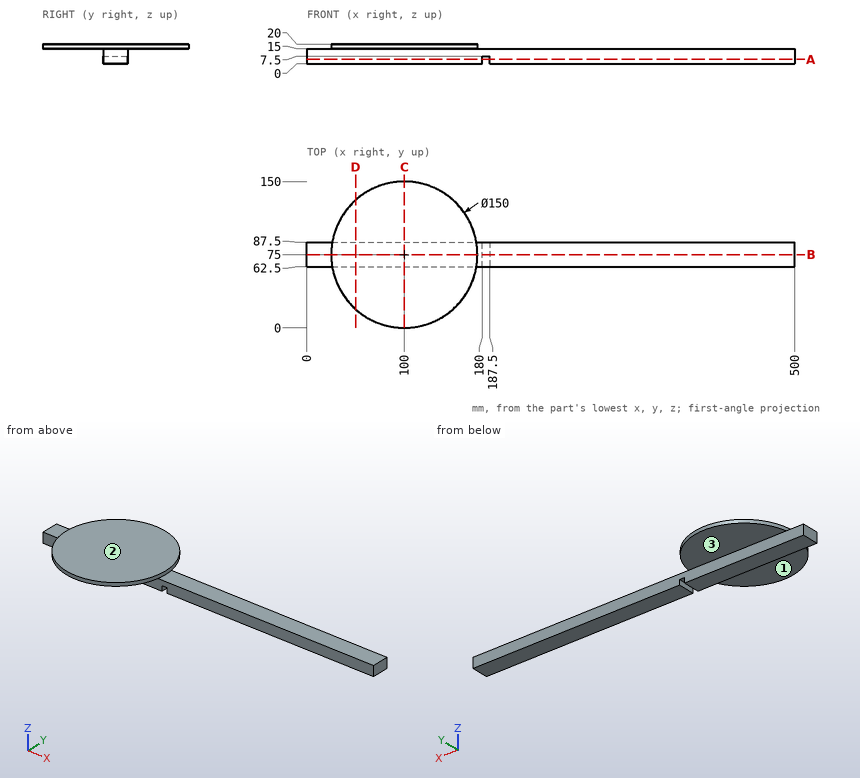
Source: three-view drawing plus pictorial views. Frame: mm from the lowest corner of the part. A direction names the side the tool comes from. Round coordinates to 2 decimals unless told otherwise and drop trailing zeros. Loops run counter-clockwise (first coordinate to the right, second up) from the corner with the lowest first, then second, coordinate; pieces in that order, holes last.
1. Section query B-B on y = 75. Output: boundary loops of the cut face in (x, z).
2. Access query for the marked faces 1, 2 and 3. Directions: +Z, -Z, +X, -X, +Y, -Y. A direction counts if a zero-diameter tool reaches every point of the face in a straight line with its end or side. Return the directions, or none.
3. Section query C-C on x = 100. Output: boundary loops of the cut face in (y, z), and give its area (4 significant figures).
4. Contact query for flat-ended pins moving along their axis: pin 1 (1 mm diameter, centred on x = 160, y = 87.5, fed in from -Z); pin 2 (7.5 mm diameter, centred on x = 10.5, y = 77.5, fed in from +Z); pin 3 (6 mm diameter, centred on x = 215.5, z = 2.5, fed in from +Y); pin 4 (6 mm diameter, centred on x = 184, y = 80, fed in from -Z). Output: stop coordinate, or through.
5. Ray query, L1, parallel to Y at x = 344, z = 10; L2, parallel to Z at x = 59.5, y = 39; L3, parallel to X at y = 66, z = 6.5. Return the intervals inside material, ascending.
6. Section query A-A on z = 4.25. Output: boundary loops of the cut face in (x, y).
7. Section query D-D on x = 50. Output: boundary loops of the cut face in (y, z).
Answers below:
1. outline: (0, 0) - (180, 0) - (180, 7.5) - (187.5, 7.5) - (187.5, 0) - (500, 0) - (500, 15) - (175, 15) - (175, 20) - (25, 20) - (25, 15) - (0, 15) - close
2. face 1: -Z, +X, -X, -Y
2. face 2: +Z, +X, -X, +Y, -Y
2. face 3: -Z, +X, -X, +Y
3. outline: (0, 15) - (62.5, 15) - (62.5, 0) - (87.5, 0) - (87.5, 15) - (150, 15) - (150, 20) - (0, 20) - close
3. area: 1,125 mm2
4. pin 1: stops at z = 0
4. pin 2: stops at z = 15
4. pin 3: stops at y = 87.5
4. pin 4: stops at z = 7.5
5. L1: y = 62.5 to 87.5
5. L2: z = 15 to 20
5. L3: x = 0 to 180, 187.5 to 500
6. outline: (0, 62.5) - (180, 62.5) - (180, 87.5) - (0, 87.5) - close; (187.5, 62.5) - (500, 62.5) - (500, 87.5) - (187.5, 87.5) - close
7. outline: (19.1, 15) - (62.5, 15) - (62.5, 0) - (87.5, 0) - (87.5, 15) - (130.9, 15) - (130.9, 20) - (19.1, 20) - close
